Part print with two shaded views. Sizes in mm from the minimum x, y, z corner. A direction names the side the tool comes from. Give positions to 0.01 mm unless a question says otherwise; leave off trailing zeros. Order: outer loops, then holes, each group sorted by start corner. A loop starts at its lowest first (then second) coordinate and runs counter-clockwise, first axis right, second up. Notation, with made-up numbers: (-20, 39) -> (-14, 39) arc R24 ccw to (-14, 73) -> close; hole circle Ø6 at (36.25, -14). An arc over 180 degrees is marked (long way). Answer as CSV lines item,"result".
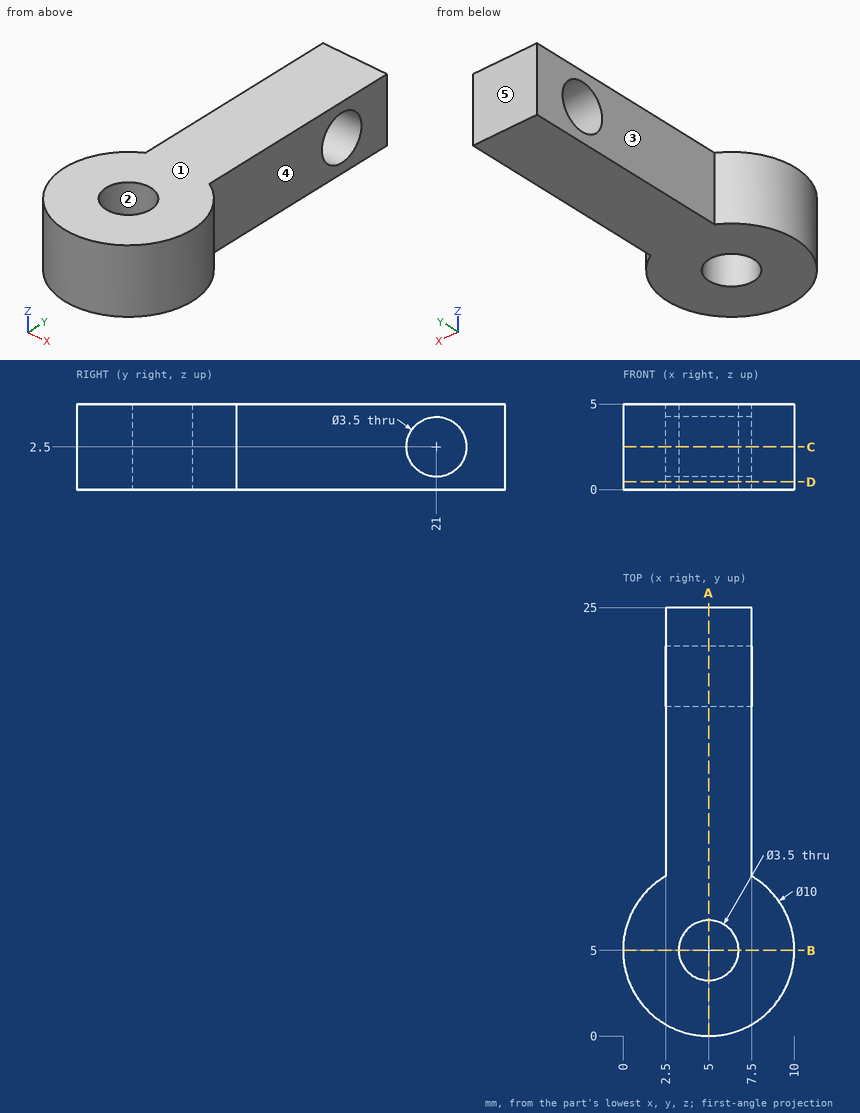
1) Band-saw the part on A-A, the plane x = 5. Write the cut outline in (y, z), then the cut area to 3 significant figures.
Data:
outline,"(0, 0) -> (3.25, 0) -> (3.25, 5) -> (0, 5) -> close; (6.75, 0) -> (25, 0) -> (25, 5) -> (6.75, 5) -> close; hole circle Ø3.5 at (21, 2.5)"
area,"97.9 mm2"
2) Pin check, flat tips, straight feed: P1, Ø5.5, axis at x = 5, y = 5, coming from the +Z side; P2, Ø2.5, axis at y = 19, z = 2.5, coming from the -X side; P3, Ø1.5, axis at y = 18.5, z = 1.5, coming from the +X side. Stop position of each tip, or through.
Data:
P1,"stops at z = 5"
P2,"stops at x = 2.5"
P3,"stops at x = 7.5"
3) Wall check: line 1 along Z through (x, y) = (4.35, 21); line 2 along Y through (x, z) = (5, 3.65); line 3 along Y through (x, z) = (5.5, 3.3). Give the ranges that are in metal, low to high. Write a range as [from, to].
Data:
line 1,"z = [0, 0.75], [4.25, 5]"
line 2,"y = [0, 3.25], [6.75, 19.68], [22.32, 25]"
line 3,"y = [0.03, 3.32], [6.68, 19.44], [22.56, 25]"
4) Which spindle directions (+Z, -Z, +X, -X, +Y, -Y) get a long thin tool onto all of the face, cutting with end or side? Do the marked faces 4 and 5. Say none if no direction does.
Data:
face 4,"+Z, -Z, +X, +Y"
face 5,"+Z, -Z, +X, -X, +Y"
5) Band-saw the part on D-D, the plane z = 0.45. Write the cut outline in (x, y), then the cut area to 3 significant figures.
Data:
outline,"(2.5, 9.33) arc R5 ccw (long way) to (7.5, 9.33) -> (7.5, 25) -> (2.5, 25) -> close; hole circle Ø3.5 at (5, 5)"
area,"145 mm2"
6) Band-saw the part on C-C, the plane z = 2.5. Write the cut outline in (x, y).
Data:
outline,"(2.5, 9.33) arc R5 ccw (long way) to (7.5, 9.33) -> (7.5, 19.25) -> (2.5, 19.25) -> close; (2.5, 22.75) -> (7.5, 22.75) -> (7.5, 25) -> (2.5, 25) -> close; hole circle Ø3.5 at (5, 5)"
7) Pull direction X, two halves, no side cores. Call the marked faces 1, 2 and 3: pulls with the +X half, pulls with the -X half, needs draft (parallel to the pull), parting line crosses it, or undercut.
Data:
face 1,"needs draft"
face 2,"undercut"
face 3,"pulls with the -X half"
8) Band-saw the part on B-B, the plane y = 5. Write the cut outline in (x, z), then the cut area to 3 significant figures.
Data:
outline,"(0, 0) -> (3.25, 0) -> (3.25, 5) -> (0, 5) -> close; (6.75, 0) -> (10, 0) -> (10, 5) -> (6.75, 5) -> close"
area,"32.5 mm2"
